Here's the drawing with two shaded views (mm, measured from the low corner). I have some questions. A direction names the side the tool comes from. Coordinates: 2 decimals unless noted, no trailing zeros. Loops run counter-clockwise (first coordinate to the right, second up) from the corner with the lowest first, then second, coordinate; pieces in that order, holes last. Notation, with made-up numbers: M 5,46 L 30,46 A14 cw 30,56 Z; hole C 37.25,-20.75 d5. An arc over 180 degrees is marked long. Return JSON: item names as keys, results as strings. Group by question number.
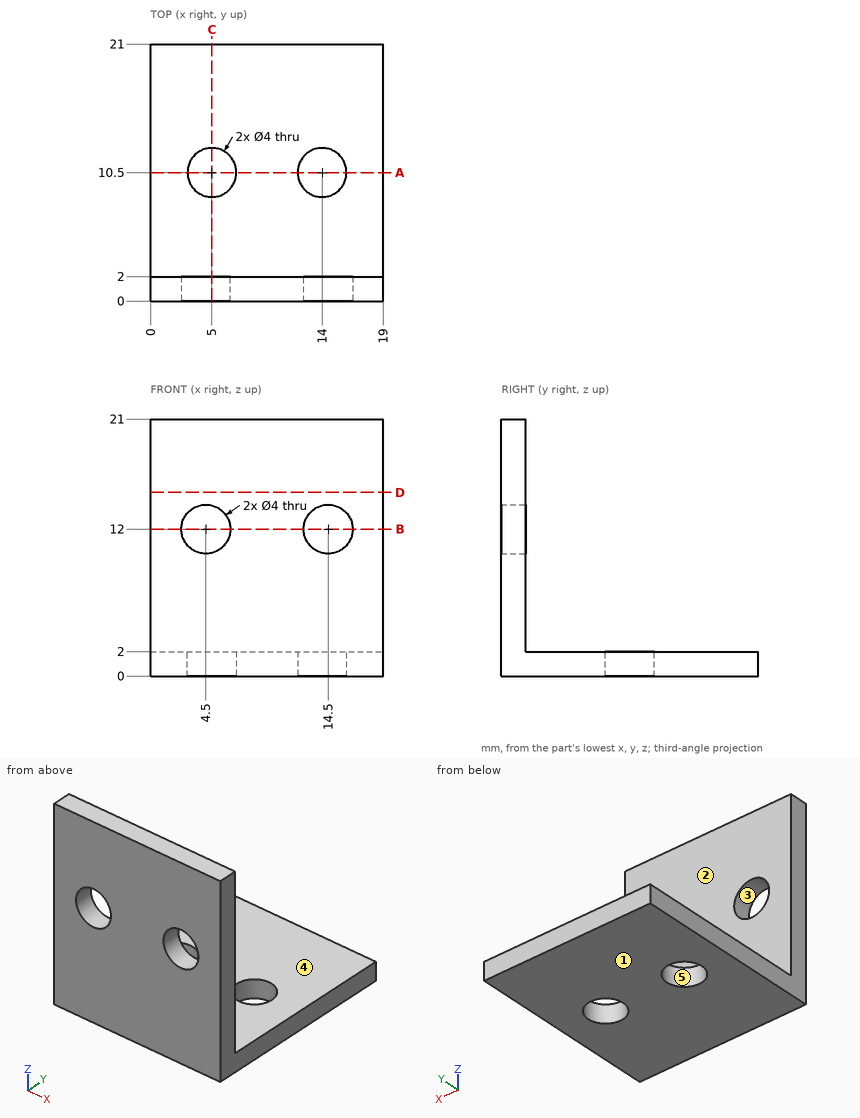
1) If we mould it in two halves opening along Z, with no side actions, what happens to the marked faces 3, 4 and 5? For each: +Z half, -Z half, draft (parallel to the pull), parting line (faces both ways), or undercut.
2) If I drill on line 1 (Y direction, x = 5, z = 1.15); line 2 (Z direction, x = 14.5, y = 1.2); line 3 (Y direction, x = 3, z = 2.5), over which ranges is the centre line in solid material (lowest first)? Write a range as from..to.
3) Suppose I cut it at B-B, the plane z = 12. List the corners of the cut face in (x, y) for me, then the cut area to 3 significant figures.
4) For the marked faces 1 and 2, which set-ups out of +Z, -Z, +X, -X, +Y, -Y let a thin tool reach every point of the face, with its end or its side?
5) Suppose I cut it at C-C, the plane x = 5. List the corners of the cut face in (y, z) for me, then the cut area to 3 significant figures.
6) Suppose I cut it at D-D, the plane z = 15. List the corners of the cut face in (x, y) for me.
7) For pin 1 (10 mm diameter, centred on x = 11, z = 10, fed in from +Y); pin 2 (5.5 mm diameter, centred on x = 11, y = 8, fed in from +Z); pin 3 (8 mm diameter, centred on y = 16.5, z = 3.5, fed in from -X); pin 4 (1 mm diameter, centred on y = 3, z = 16, fed in from +X), each with a flat end and sliding along its axis, tell me the tip position at first contact or that it passes through.
8) Suppose I cut it at A-A, the plane y = 10.5. List the corners of the cut face in (x, z) for me.
Returned:
{
 "1": {"face 3": "undercut", "face 4": "+Z half", "face 5": "draft"},
 "2": {"line 1": "y = 0..8.5, 12.5..21", "line 2": "z = 0..10, 14..21", "line 3": "y = 0..2"},
 "3": {"outline": "M 0,0 L 2.5,0 L 2.5,2 L 0,2 Z; M 6.5,0 L 12.5,0 L 12.5,2 L 6.5,2 Z; M 16.5,0 L 19,0 L 19,2 L 16.5,2 Z", "area": "22.0 mm²"},
 "4": {"face 1": "-Z, +X, -X, +Y, -Y", "face 2": "+Z, +X, -X, +Y"},
 "5": {"outline": "M 0,0 L 8.5,0 L 8.5,2 L 2,2 L 2,10.06 L 0,10.06 Z; M 0,13.94 L 2,13.94 L 2,21 L 0,21 Z; M 12.5,0 L 21,0 L 21,2 L 12.5,2 Z", "area": "64.3 mm²"},
 "6": {"outline": "M 0,0 L 19,0 L 19,2 L 0,2 Z"},
 "7": {"pin 1": "stops at y = 2", "pin 2": "stops at z = 2", "pin 3": "stops at x = 0", "pin 4": "passes through"},
 "8": {"outline": "M 0,0 L 3,0 L 3,2 L 0,2 Z; M 7,0 L 12,0 L 12,2 L 7,2 Z; M 16,0 L 19,0 L 19,2 L 16,2 Z"}
}
